Check sheet for the modelled part. Datum: model origin and axes. Units: mm. A direction names the side the tool comes from. Round coordinates to 2 decimals unless told otherwise and drop trailing zeros. Order: outer loops, then holes, each group sorted by start corner. A loop starts at its lowest first (then second) coordinate and runs counter-clockwise, first axis right, second up. Notation, with made-up numbers: (-32, 15.5) -> (15, 15.5) arc R12 ccw to (15, 23.5) -> close; hole circle Ø9 at (-9, 57). An arc over 180 degrees is marked (long way). Use CSV: the item, a comma, the result in double quotes.
```python
from build123d import *

# Parameters (mm, degrees)
SKETCH1_R           = 1.5
SKETCH1_R_2         = 2.5
BOSS_EXTRUDE1_DEPTH = 3
CUT_EXTRUDE1_DEPTH  = 3
FILLET1_R           = 3
CHAMFER4_SIZE       = 15
CHAMFER5_SIZE       = 10
SKETCH13_W          = 30
SKETCH13_H          = 8
BOSS_EXTRUDE5_DEPTH = 3
SKETCH8_W           = 95
SKETCH8_H           = 65.304735008
CUT_EXTRUDE5_DEPTH  = 10
SKETCH11_W          = 95
SKETCH11_H          = 7
BOSS_EXTRUDE3_DEPTH = 3
SKETCH10_R          = 1.5
CUT_EXTRUDE6_DEPTH  = 3
BOSS_EXTRUDE4_DEPTH = 3
CHAMFER6_SIZE       = 8
SKETCH17_R          = 2
CUT_EXTRUDE9_DEPTH  = 10
SKETCH15_W          = 40
SKETCH15_H          = 3
CUT_EXTRUDE8_DEPTH  = 10
BOSS_EXTRUDE6_START = -3
BOSS_EXTRUDE6_DEPTH = 3
SKETCH18_W          = 5
SKETCH18_H          = 3
CUT_EXTRUDE11_DEPTH = 10


with BuildPart() as part:
    # Sketch1 → Boss-Extrude1 (new body)
    with BuildSketch(Plane.XY):
        with BuildLine():
            Line((40.5, -40), (44.5, -40))
            Line((44.5, -40), (47.5, -37))
            Line((47.5, -37), (47.5, 10))
            Line((47.5, 10), (47.5, 15))
            Line((47.5, 15), (52.5, 15))
            Line((52.5, 15), (70, 15))
            ThreePointArc((70, 15), (73.535533906, 16.464466094), (75, 20))
            Line((75, 20), (75, 60))
            ThreePointArc((75, 60), (73.535533906, 63.535533906), (70, 65))
            Line((70, 65), (-70, 65))
            ThreePointArc((-70, 65), (-73.535533906, 63.535533906), (-75, 60))
            Line((-75, 60), (-75, 20))
            ThreePointArc((-75, 20), (-73.535533906, 16.464466094), (-70, 15))
            Line((-70, 15), (-52.5, 15))
            Line((-52.5, 15), (-47.5, 15))
            Line((-47.5, 15), (-47.5, 10))
            Line((-47.5, 10), (-47.5, -37))
            Line((-47.5, -37), (-44.5, -40))
            Line((-44.5, -40), (-40.5, -40))
            Line((-40.5, -40), (-37.5, -37))
            Line((-37.5, -37), (-37.5, 10))
            ThreePointArc((-37.5, 10), (-36.035533906, 13.535533906), (-32.5, 15))
            Line((-32.5, 15), (32.5, 15))
            ThreePointArc((32.5, 15), (36.035533906, 13.535533906), (37.5, 10))
            Line((37.5, 10), (37.5, -37))
            Line((37.5, -37), (40.5, -40))
        make_face()
        with Locations((-42.5, -20)):
            Circle(SKETCH1_R, mode=Mode.SUBTRACT)
        with Locations((-42.5, -35)):
            Circle(SKETCH1_R, mode=Mode.SUBTRACT)
        with Locations((42.5, -20)):
            Circle(SKETCH1_R, mode=Mode.SUBTRACT)
        with Locations((42.5, -35)):
            Circle(SKETCH1_R, mode=Mode.SUBTRACT)
        with Locations((60, 40)):
            Circle(SKETCH1_R_2, mode=Mode.SUBTRACT)
        with Locations((15, 60)):
            Circle(SKETCH1_R, mode=Mode.SUBTRACT)
        with Locations(Location((-15, 60, 0), (0, 0, 180))):
            Circle(SKETCH1_R, mode=Mode.SUBTRACT)
        with Locations(Location((-60, 40, 0), (0, 0, 180))):
            Circle(SKETCH1_R_2, mode=Mode.SUBTRACT)
    extrude(amount=BOSS_EXTRUDE1_DEPTH)

    # Sketch3 → Cut-Extrude1 (cut)
    with BuildSketch(Plane.XY.offset(3)):
        Polygon((65, 50), (65, 30), (47.5, 30), (47.5, 15), (75, 15), (75, 23.034767996), (75, 32.364095159), (75, 65), (47.5, 65), (47.5, 50), align=None)
        Polygon((-47.5, 65), (-75, 65), (-75, 32.364095159), (-75, 23.034767996), (-75, 15), (-47.5, 15), (-47.5, 30), (-65, 30), (-65, 50), (-47.5, 50), align=None)
    extrude(amount=-CUT_EXTRUDE1_DEPTH, mode=Mode.SUBTRACT)

    # Fillet1
    fillet1_edges = [part.edges().sort_by_distance(p)[0] for p in [
        (65, 50, 1.5),
        (65, 30, 1.5),
        (-65, 50, 1.5),
        (-65, 30, 1.5),
    ]]
    fillet(fillet1_edges, radius=FILLET1_R)

    # Chamfer4
    chamfer4_edges = [part.edges().sort_by_distance(p)[0] for p in [
        (47.5, 65, 1.5),
        (-47.5, 65, 1.5),
    ]]
    chamfer(chamfer4_edges, length=CHAMFER4_SIZE - 0.0001)  # a hair under: the kernel refuses the full size

    # Chamfer5
    chamfer5_edges = [part.edges().sort_by_distance(p)[0] for p in [
        (47.5, 30, 1.5),
        (-47.5, 30, 1.5),
    ]]
    chamfer(chamfer5_edges, length=CHAMFER5_SIZE)

    # Sketch13 → Boss-Extrude5 (add)
    with BuildSketch(Plane.XY.offset(3)):
        with Locations((0, 69)):
            Rectangle(SKETCH13_W, SKETCH13_H)
    extrude(amount=-BOSS_EXTRUDE5_DEPTH)

    # Sketch8 → Cut-Extrude5 (cut)
    with BuildSketch(Plane.XY.offset(3)):
        with Locations((0, -12.652367504)):
            Rectangle(SKETCH8_W, SKETCH8_H)
    extrude(amount=-CUT_EXTRUDE5_DEPTH, mode=Mode.SUBTRACT)

    # Sketch11 → Boss-Extrude3 (add)
    with BuildSketch(Plane.XY.offset(3)):
        with Locations((0, 16.5)):
            Rectangle(SKETCH11_W, SKETCH11_H)
    extrude(amount=-BOSS_EXTRUDE3_DEPTH)

    # Sketch10 → Cut-Extrude6 (cut)
    with BuildSketch(Plane.XY.offset(3)):
        with Locations((5, 67.89)):
            Circle(SKETCH10_R)
        with Locations(Location((-5, 67.89, 0), (0, 0, 180))):
            Circle(SKETCH10_R)
        with Locations((-5, 18.11)):
            Circle(SKETCH10_R)
        with Locations(Location((5, 18.11, 0), (0, 0, 180))):
            Circle(SKETCH10_R)
        Polygon((-30, 13), (-28, 15), (28, 15), (30, 13), align=None)
    extrude(amount=-CUT_EXTRUDE6_DEPTH, mode=Mode.SUBTRACT)

    # Sketch12 → Boss-Extrude4 (add)
    with BuildSketch(Plane.XY.offset(3)):
        Polygon((47.5, 13), (47.5, -12), (35.5, -12), (35.5, 7.5), (30, 13), (35.5, 13), align=None)
        Polygon((-35.5, 13), (-47.5, 13), (-47.5, -12), (-35.5, -12), (-35.5, 7.5), (-30, 13), align=None)
    extrude(amount=-BOSS_EXTRUDE4_DEPTH)

    # Chamfer6
    chamfer6_edges = [part.edges().sort_by_distance(p)[0] for p in [
        (15, 65, 1.5),
        (-15, 65, 1.5),
    ]]
    chamfer(chamfer6_edges, length=CHAMFER6_SIZE - 0.0001)  # a hair under: the kernel refuses the full size

    # Sketch17 → Cut-Extrude9 (cut)
    with BuildSketch(Plane(origin=(0, 0, 0), x_dir=(-1, 0, 0), z_dir=(0, 0, -1))):
        with Locations((-28.88804467, 50.488766948)):
            Circle(SKETCH17_R)
        with Locations((-28.88804467, 30.407216077)):
            Circle(SKETCH17_R)
        with Locations((31.126767325, 30.407216077)):
            Circle(SKETCH17_R)
        with Locations((31.126767325, 50.488766948)):
            Circle(SKETCH17_R)
    extrude(amount=-CUT_EXTRUDE9_DEPTH, mode=Mode.SUBTRACT)

    # Sketch15 → Cut-Extrude8 (cut)
    with BuildSketch(Plane(origin=(0, 0, 0), x_dir=(-1, 0, 0), z_dir=(0, 0, -1))):
        with Locations((0, 20.5)):
            Rectangle(SKETCH15_W, SKETCH15_H)
    extrude(amount=-CUT_EXTRUDE8_DEPTH, mode=Mode.SUBTRACT)

    # Sketch16 → Boss-Extrude6 (add)
    with BuildSketch(Plane(origin=(0, 0, 0), x_dir=(-1, 0, 0), z_dir=(0, 0, -1)).offset(BOSS_EXTRUDE6_START)):
        with BuildLine():
            Line((3.792564702, 19), (6.207435298, 19))
            ThreePointArc((6.207435298, 19), (5, 16.61), (3.792564702, 19))
        make_face()
        with BuildLine():
            Line((-6.207435298, 19), (-3.792564702, 19))
            ThreePointArc((-3.792564702, 19), (-5, 16.61), (-6.207435298, 19))
        make_face()
    extrude(amount=BOSS_EXTRUDE6_DEPTH)

    # Sketch18 → Cut-Extrude11 (cut)
    with BuildSketch(Plane(origin=(0, 0, 0), x_dir=(-1, 0, 0), z_dir=(0, 0, -1))):
        with Locations((-131.776111861, 19.947341704)):
            Rectangle(SKETCH18_W, SKETCH18_H)
        with Locations((-41.5, -7.5)):
            Rectangle(SKETCH18_W, SKETCH18_H)
        with Locations((41.5, -7.5)):
            Rectangle(SKETCH18_W, SKETCH18_H)
    extrude(amount=-CUT_EXTRUDE11_DEPTH, mode=Mode.SUBTRACT)


solid = part.part
```
Q1. Sectioned sample at C-C, the plane x = 25. Enter the section's corners in (y, z), then the cut area to 3 significant figures.
Result sheet:
outline,"(15, 0) -> (65, 0) -> (65, 3) -> (15, 3) -> close"
area,"150 mm^2"
Q2. Sectioned sample at B-B, the plane x = -1.5. Enter the section's corners in (y, z).
Result sheet:
outline,"(15, 0) -> (19, 0) -> (19, 3) -> (15, 3) -> close; (22, 0) -> (73, 0) -> (73, 3) -> (22, 3) -> close"
Q3. Go/stop test with flat-tipped pins: pin 1 (1.5 mm diameter, centred on x = 50, z = 0.5, fed in from +Y); pin 2 (0.9 mm diameter, centred on y = 21, z = 1, fed in from -X); pin 3 (0.9 mm diameter, centred on y = -8, z = 1, fed in from -X); pin 4 (3 mm diameter, centred on x = 28.89, y = 50.49, fed in from +Z). Record where each tip stops, or that it passes through.
Result sheet:
pin 1,"stops at y = 50"
pin 2,"stops at x = -48.95"
pin 3,"stops at x = -47.5"
pin 4,"passes through"
Q4. Scan lines: L1, parallel to X at y = -7.5, z = 2.75; L2, parallel to Y at x = 15, z = 0.95; L3, parallel to Y at x = 5, z = 1.4. Record each from-to range of solid material in increasing order.
Result sheet:
L1,"x = -47.5 to -44, -39 to -35.5, 35.5 to 39, 44 to 47.5"
L2,"y = 15 to 19, 22 to 58.5, 61.5 to 73"
L3,"y = 15 to 19, 22 to 66.39, 69.39 to 73"
Q5. Sectioned sample at D-D, the plane z = 1.55. State how many separate pieces and enclosed holes the cut face has, then the cut area to 3 significant figures.
Result sheet:
separate pieces,"1"
enclosed holes,"13"
area,"6,060 mm^2"
Q6. Sectioned sample at A-A, the plane y = 40. Enter the section's corners in (x, z), then the cut area to 3 significant figures.
Result sheet:
outline,"(-65, 0) -> (-62.5, 0) -> (-62.5, 3) -> (-65, 3) -> close; (-57.5, 0) -> (57.5, 0) -> (57.5, 3) -> (-57.5, 3) -> close; (62.5, 0) -> (65, 0) -> (65, 3) -> (62.5, 3) -> close"
area,"360 mm^2"
Q7. Mould release check, pull along Y, two halves, no side actions. Record for faces 1 (the face through (-64.1, 30.86, 1.48)), 2 (the face through (-19, 69, 2)), 3 (the face through (44, -8, 1)): pulls with the +Y half, pulls with the -Y half, needs draft (parallel to the pull), parting line crosses it, or undercut.
Result sheet:
face 1,"pulls with the -Y half"
face 2,"pulls with the +Y half"
face 3,"undercut"
Q8. Access from +Z, -Z, +X, -X, +Y, -Y to the whole of each face (thin tool, end or side, straight path). Record for faces 4 (the face through (39, -8, 1)), 5 (the face through (60, 30, 2)), 6 (the face through (28, 65, 1)), 7 (the face through (-32, 11, 2)).
Result sheet:
face 4,"+Z, -Z"
face 5,"+Z, -Z, +X, -Y"
face 6,"+Z, -Z, +X, +Y"
face 7,"+Z, -Z, -Y"
